```python
from build123d import *

# Parameters (mm, degrees)
SALIENTE_EXTRUIR1_DEPTH      = 7
SALIENTE_EXTRUIR1_DEPTH_BACK = 7
REDONDEO1_R                  = 0.4
SALIENTE_EXTRUIR2_DEPTH      = 1.5
SALIENTE_EXTRUIR2_DEPTH_BACK = 1.5
CORTAR_EXTRUIR1_REACH        = 5
CROQUIS4_R                   = 1
CROQUIS5_R                   = 1
CORTAR_EXTRUIR2_DEPTH        = 8.5


with BuildPart() as part:
    # Croquis2 → Saliente-Extruir1 (new body, two sides)
    with BuildSketch(Plane.XY) as saliente_extruir1_sk:
        with BuildLine():
            Line((-10, 0), (-10, -11.6))
            ThreePointArc((-10, -11.6), (-10.117157288, -11.882842712), (-10.4, -12))
            Line((-10.4, -12), (-14, -12))
            Line((-14, -12), (-14, -15))
            Line((-14, -15), (-7.4, -15))
            Line((-7.4, -15), (-7.4, -14.6))
            Line((-7.4, -14.6), (-7, -14.6))
            Line((-7, -14.6), (-7, -7.141428429))
            ThreePointArc((-7, -7.141428429), (0, -10), (7, -7.141428429))
            Line((7, -7.141428429), (7, -14.6))
            Line((7, -14.6), (7.4, -14.6))
            Line((7.4, -14.6), (7.4, -15))
            Line((7.4, -15), (14, -15))
            Line((14, -15), (14, -12))
            Line((14, -12), (10.4, -12))
            ThreePointArc((10.4, -12), (10.117157288, -11.882842712), (10, -11.6))
            Line((10, -11.6), (10, 0))
            ThreePointArc((10, 0), (8.215838363, 5.700877125), (3.5, 9.367496998))
            Line((3.5, 9.367496998), (3.5, 12.967496998))
            Line((3.5, 12.967496998), (0.5, 12.967496998))
            Line((0.5, 12.967496998), (0.5, 9.987492178))
            Line((0.5, 9.987492178), (0.5, 6.982120022))
            ThreePointArc((0.5, 6.982120022), (0, -7), (-0.5, 6.982120022))
            Line((-0.5, 6.982120022), (-0.5, 9.987492178))
            Line((-0.5, 9.987492178), (-0.5, 12.967496998))
            Line((-0.5, 12.967496998), (-3.5, 12.967496998))
            Line((-3.5, 12.967496998), (-3.5, 9.367496998))
            ThreePointArc((-3.5, 9.367496998), (-8.215838363, 5.700877125), (-10, 0))
        make_face()
    extrude(amount=SALIENTE_EXTRUIR1_DEPTH)
    extrude(saliente_extruir1_sk.sketch, amount=-SALIENTE_EXTRUIR1_DEPTH_BACK)

    # Redondeo1
    redondeo1_edges = [part.edges().sort_by_distance(p)[0] for p in [
        (-2, 12.967496998, -7),
        (2, 12.967496998, -7),
        (2, 12.967496998, 7),
        (-2, 12.967496998, 7),
    ]]
    fillet(redondeo1_edges, radius=REDONDEO1_R)

    # Croquis3 → Saliente-Extruir2 (add, two sides)
    with BuildSketch(Plane.XY) as saliente_extruir2_sk:
        Polygon((10, 0), (14, -12), (10, -12), align=None)
        Polygon((-10, -12), (-14, -12), (-10, 0), align=None)
    extrude(amount=SALIENTE_EXTRUIR2_DEPTH)
    extrude(saliente_extruir2_sk.sketch, amount=-SALIENTE_EXTRUIR2_DEPTH_BACK)

    # Croquis4 → Cortar-Extruir1 (cut, up to next)
    with BuildSketch(Plane(origin=(0, -12, 0), x_dir=(1, 0, 0), z_dir=(0, 1, 0)), mode=Mode.PRIVATE) as cortar_extruir1_sk1:
        with Locations((12, -4.2)):
            Circle(CROQUIS4_R)
    cortar_extruir1_tool1 = extrude(cortar_extruir1_sk1.sketch, amount=-CORTAR_EXTRUIR1_REACH, mode=Mode.PRIVATE) & part.part
    add(cortar_extruir1_tool1.solids().sort_by_distance((12, -12, 4.2))[0], mode=Mode.SUBTRACT)
    # Croquis4 → Cortar-Extruir1 (cut, up to next)
    with BuildSketch(Plane(origin=(0, -12, 0), x_dir=(1, 0, 0), z_dir=(0, 1, 0)), mode=Mode.PRIVATE) as cortar_extruir1_sk2:
        with Locations((12, 4.2)):
            Circle(CROQUIS4_R)
    cortar_extruir1_tool2 = extrude(cortar_extruir1_sk2.sketch, amount=-CORTAR_EXTRUIR1_REACH, mode=Mode.PRIVATE) & part.part
    add(cortar_extruir1_tool2.solids().sort_by_distance((12, -12, -4.2))[0], mode=Mode.SUBTRACT)
    # Croquis4 → Cortar-Extruir1 (cut, up to next)
    with BuildSketch(Plane(origin=(0, -12, 0), x_dir=(1, 0, 0), z_dir=(0, 1, 0)), mode=Mode.PRIVATE) as cortar_extruir1_sk3:
        with Locations((-12, 4.2)):
            Circle(CROQUIS4_R)
    cortar_extruir1_tool3 = extrude(cortar_extruir1_sk3.sketch, amount=-CORTAR_EXTRUIR1_REACH, mode=Mode.PRIVATE) & part.part
    add(cortar_extruir1_tool3.solids().sort_by_distance((-12, -12, -4.2))[0], mode=Mode.SUBTRACT)
    # Croquis4 → Cortar-Extruir1 (cut, up to next)
    with BuildSketch(Plane(origin=(0, -12, 0), x_dir=(1, 0, 0), z_dir=(0, 1, 0)), mode=Mode.PRIVATE) as cortar_extruir1_sk4:
        with Locations((-12, -4.2)):
            Circle(CROQUIS4_R)
    cortar_extruir1_tool4 = extrude(cortar_extruir1_sk4.sketch, amount=-CORTAR_EXTRUIR1_REACH, mode=Mode.PRIVATE) & part.part
    add(cortar_extruir1_tool4.solids().sort_by_distance((-12, -12, 4.2))[0], mode=Mode.SUBTRACT)

    # Croquis5 → Cortar-Extruir2 (cut)
    with BuildSketch(Plane(origin=(3.5, 0, 0), x_dir=(0, 0, -1), z_dir=(1, 0, 0))):
        with Locations((0, 11.167496998)):
            Circle(CROQUIS5_R)
        with Locations((4, 11.167496998)):
            Circle(CROQUIS5_R)
        with Locations((-4, 11.167496998)):
            Circle(CROQUIS5_R)
    extrude(amount=-CORTAR_EXTRUIR2_DEPTH, mode=Mode.SUBTRACT)


solid = part.part
```
Could you check a few things on this model? Use its own coordinates, in mm. A direction names the side the tool comes from. Coordinates: 2 decimals unless noted, no trailing zeros. Write each loop counter-clockwise with the first axis right and the second up, starting at its lowest first coordinate (ties: lowest second). Pieces come first, ordered by that corner, then holes. Notation, with made-up numbers: (0, 49.25) -> (43, 49.25) arc R14 ccw to (43, 76.25) -> close; hole circle Ø8 at (21, 4.25). An arc over 180 degrees is marked (long way). Return JSON: item names as keys, results as strings.
(1) I'm going to push flat-ended pins straight in: pin 1 (3 mm diameter, centred on y = -2.5, z = -1, fed in from +X); pin 2 (1.8 mm diameter, centred on x = -11.5, z = -5, fed in from +Y); pin 3 (5 mm diameter, centred on x = -1.5, z = 0.5, fed in from -Y); pin 4 (1.6 mm diameter, centred on y = 11.17, z = 4, fed in from -X). Where does each tip first touch, or does it pass through?
Numbers:
{"pin 1": "stops at x = 11.33", "pin 2": "stops at y = -12", "pin 3": "stops at y = -10", "pin 4": "passes through"}
(2) Imagine slicing it at B-B, the plane x = -12. Please give me the cut outline in (y, z).
Numbers:
{"outline": "(-15, -7) -> (-12, -7) -> (-12, -5.2) -> (-15, -5.2) -> close; (-15, -3.2) -> (-12, -3.2) -> (-12, -1.5) -> (-6, -1.5) -> (-6, 1.5) -> (-12, 1.5) -> (-12, 3.2) -> (-15, 3.2) -> close; (-15, 5.2) -> (-12, 5.2) -> (-12, 7) -> (-15, 7) -> close"}
(3) Which directions (+Z, -Z, +X, -X, +Y, -Y) give clear straight access to the entire face, cutting with the end or side of a thin tool? Please do faces 1 (the flat face through (0.5, 10, 0)), 2 (the flat face through (3.5, 10, 0)), 3 (the flat face through (-11, -9, 1.5)).
Numbers:
{"face 1": "+Z, -Z, +Y", "face 2": "+Z, -Z, +X, +Y", "face 3": "+Z, -X, +Y"}
(4) Imagine slicing it at C-C, the plane y = 5.5. Please give me the cut outline in (x, z).
Numbers:
{"outline": "(-8.35, -7) -> (-4.33, -7) -> (-4.33, 7) -> (-8.35, 7) -> close; (4.33, -7) -> (8.35, -7) -> (8.35, 7) -> (4.33, 7) -> close"}
(5) Imagine slicing it at D-D, the plane z = 2.25. Please give me the cut outline in (x, y), then the cut area to 3 significant figures.
Numbers:
{"outline": "(-14, -15) -> (-7.4, -15) -> (-7.4, -14.6) -> (-7, -14.6) -> (-7, -7.14) arc R10 ccw to (7, -7.14) -> (7, -14.6) -> (7.4, -14.6) -> (7.4, -15) -> (14, -15) -> (14, -12) -> (10.4, -12) arc R0.4 cw to (10, -11.6) -> (10, 0) arc R10 ccw to (3.5, 9.37) -> (3.5, 12.97) -> (0.5, 12.97) -> (0.5, 6.98) arc R7 cw (long way) to (-0.5, 6.98) -> (-0.5, 12.97) -> (-3.5, 12.97) -> (-3.5, 9.37) arc R10 ccw to (-10, 0) -> (-10, -11.6) arc R0.4 cw to (-10.4, -12) -> (-14, -12) -> close", "area": "261 mm2"}
(6) We'd pull the mould along Z, two halves only. Please class faces 4 (the flat face through (14, -14, 0)), 5 (the cylindrical face through (2.02, 12.16, 4.13)), 6 (the flat face through (11, -9, -1.5)): +Z half, -Z half, draft (parallel to the pull), parting line (faces both ways), or undercut.
Numbers:
{"face 4": "draft", "face 5": "undercut", "face 6": "-Z half"}
(7) Imagine slicing it at A-A, the plane x = -1. Please give me the cut outline in (y, z).
Numbers:
{"outline": "(-9.95, -7) -> (-6.93, -7) -> (-6.93, 7) -> (-9.95, 7) -> close; (6.93, -7) -> (12.57, -7) arc R0.4 ccw to (12.97, -6.6) -> (12.97, 6.6) arc R0.4 ccw to (12.57, 7) -> (6.93, 7) -> close; hole circle Ø2 at (11.17, -4); hole circle Ø2 at (11.17, 0); hole circle Ø2 at (11.17, 4)"}
(8) I need wall thicknesses on L1, parallel to Z at x = 12, y = -13.1; L2, parallel to X at y = 10, z = -4.25; L3, parallel to X at y = -13.05, z = -4.2. Which ranges of each line are inside material? Lowest first, please.
Numbers:
{"L1": "z = -7 to -5.2, -3.2 to 3.2, 5.2 to 7", "L2": "x = -3.5 to -0.5, 0.5 to 3.5", "L3": "x = -14 to -13, -11 to -7, 7 to 11, 13 to 14"}
